Verification items for the finished model (mm, model axes). A direction names the side the tool comes from. Give positions to 0.01 mm unless a question says otherwise; leave off trailing zeros. Loops run counter-clockwise (first coordinate to the right, second up) from the corner with the lowest first, then second, coordinate; pieces in that order, holes last. Notation, with made-up numbers: (-10.5, -9) - (33.5, -9) arc R23 cw to (33.5, 9) - close; hole circle Ø5 at (-24.5, -1.5). An arc over 180 degrees is marked (long way). Use one line per item in the form item = value.
```python
from build123d import *

# Parameters (mm, degrees)
BOSS_EXTRUDE1_DEPTH                        = 1.6
CHAMFER1_SIZE                              = 3
BOSS_EXTRUDE2_DEPTH                        = 11
CHAMFER2_SIZE                              = 3
FILLET1_R                                  = 2
SKETCH3_R                                  = 1
CUT_EXTRUDE1_DEPTH                         = 11
SKETCH4_R                                  = 1.05
CUT_EXTRUDE2_DEPTH                         = 13.6
SKETCH5_R                                  = 1
CUT_EXTRUDE3_DEPTH                         = 2.6
MIRROR1_AT_THE_SECOND_PLANE_COPY_1_SKETC_R = 1
MIRROR1_AT_THE_SECOND_PLANE_COPY_1_DEPTH   = 11
MIRROR1_AT_THE_SECOND_PLANE_COPY_2_SKETC_R = 1.05
MIRROR1_AT_THE_SECOND_PLANE_COPY_2_DEPTH   = 13.6
MIRROR1_AT_THE_SECOND_PLANE_COPY_3_SKETC_R = 1
MIRROR1_AT_THE_SECOND_PLANE_COPY_3_DEPTH   = 2.6
SKETCH6_W                                  = 8.5
SKETCH6_H                                  = 7
BOSS_EXTRUDE3_DEPTH                        = 3.3
SKETCH7_R                                  = 0.5
SKETCH7_R_2                                = 1
CUT_EXTRUDE4_DEPTH                         = 2.6
LPATTERN1_COUNT                            = 3
LPATTERN1_PITCH                            = 2.54
LPATTERN1_COL_COUNT                        = 3
LPATTERN1_COL_PITCH                        = 2.54


with BuildPart() as part:
    # Sketch1 → Boss-Extrude1 (new body)
    with BuildSketch(Plane(origin=(0, 0, 0), x_dir=(1, 0, 0), z_dir=(0, 1, 0))):
        Polygon((-17, 20), (-17, -20), (17, -20), align=None)
        Polygon((17, 20), (17, -20), (-17, 20), align=None)
    extrude(amount=BOSS_EXTRUDE1_DEPTH)

    # Chamfer1
    chamfer1_edges = [part.edges().sort_by_distance(p)[0] for p in [
        (-17, 0.8, -20),
        (17, 0.8, -20),
        (17, 0.8, 20),
        (-17, 0.8, 20),
    ]]
    chamfer(chamfer1_edges, length=CHAMFER1_SIZE)

    # Sketch2 → Boss-Extrude2 (add)
    with BuildSketch(Plane(origin=(0, 1.6, 0), x_dir=(1, 0, 0), z_dir=(0, 1, 0))):
        Polygon((-15, 13), (15, 13), (15, -13), align=None)
        Polygon((-15, 13), (15, -13), (-15, -13), align=None)
    extrude(amount=BOSS_EXTRUDE2_DEPTH)

    # Chamfer2
    chamfer2_edges = [part.edges().sort_by_distance(p)[0] for p in [
        (15, 7.1, -13),
        (-15, 7.1, -13),
        (-15, 7.1, 13),
        (15, 7.1, 13),
    ]]
    chamfer(chamfer2_edges, length=CHAMFER2_SIZE)

    # Fillet1
    fillet1_edges = [part.edges().sort_by_distance(p)[0] for p in [
        (-15, 7.1, 10),
        (-15, 7.1, -10),
        (12, 7.1, -13),
        (-12, 7.1, -13),
        (15, 7.1, 10),
        (15, 7.1, -10),
        (-12, 7.1, 13),
        (12, 7.1, 13),
    ]]
    fillet(fillet1_edges, radius=FILLET1_R)

    # Sketch3 → Cut-Extrude1 (cut)
    with BuildSketch(Plane(origin=(0, 12.6, 0), x_dir=(1, 0, 0), z_dir=(0, 1, 0))):
        with Locations((-11.378679656, 9.378679656)):
            Circle(SKETCH3_R)
    cut_extrude1 = extrude(amount=-CUT_EXTRUDE1_DEPTH, mode=Mode.SUBTRACT)

    # Sketch4 → Cut-Extrude2 (cut, through all)
    with BuildSketch(Plane(origin=(0, 12.6, 0), x_dir=(1, 0, 0), z_dir=(0, 1, 0))):
        with Locations((15, 15.5)):
            Circle(SKETCH4_R)
    cut_extrude2 = extrude(amount=-CUT_EXTRUDE2_DEPTH, mode=Mode.SUBTRACT)

    # Sketch5 → Cut-Extrude3 (cut, through all)
    with BuildSketch(Plane(origin=(0, 1.6, 0), x_dir=(1, 0, 0), z_dir=(0, 1, 0))):
        with Locations((-12.35, 20)):
            Circle(SKETCH5_R)
    cut_extrude3 = extrude(amount=-CUT_EXTRUDE3_DEPTH, mode=Mode.SUBTRACT)

    # Mirror1: Cut-Extrude1, Cut-Extrude2, Cut-Extrude3 across plane
    add(cut_extrude1.mirror(Plane.XY), mode=Mode.SUBTRACT)
    add(cut_extrude2.mirror(Plane.XY), mode=Mode.SUBTRACT)
    add(cut_extrude3.mirror(Plane.XY), mode=Mode.SUBTRACT)

    # Mirror1 at the second plane: Cut-Extrude3, Cut-Extrude1, Cut-Extrude2 across plane
    add(cut_extrude3.mirror(Plane(origin=(0, 0, 0), x_dir=(0, 0, 1), z_dir=(1, 0, 0))), mode=Mode.SUBTRACT)
    add(cut_extrude1.mirror(Plane(origin=(0, 0, 0), x_dir=(0, 0, 1), z_dir=(1, 0, 0))), mode=Mode.SUBTRACT)
    add(cut_extrude2.mirror(Plane(origin=(0, 0, 0), x_dir=(0, 0, 1), z_dir=(1, 0, 0))), mode=Mode.SUBTRACT)

    # Mirror1 at the second plane copy 1 sketc → Mirror1 at the second plane copy 1 (cut)
    with BuildSketch(Plane(origin=(0, 12.6, 0), x_dir=(-1, 0, 0), z_dir=(0, 1, 0))):
        with Locations((-11.378679656, 9.378679656)):
            Circle(MIRROR1_AT_THE_SECOND_PLANE_COPY_1_SKETC_R)
    extrude(amount=-MIRROR1_AT_THE_SECOND_PLANE_COPY_1_DEPTH, mode=Mode.SUBTRACT)

    # Mirror1 at the second plane copy 2 sketc → Mirror1 at the second plane copy 2 (cut, through all)
    with BuildSketch(Plane(origin=(0, 12.6, 0), x_dir=(-1, 0, 0), z_dir=(0, 1, 0))):
        with Locations((15, 15.5)):
            Circle(MIRROR1_AT_THE_SECOND_PLANE_COPY_2_SKETC_R)
    extrude(amount=-MIRROR1_AT_THE_SECOND_PLANE_COPY_2_DEPTH, mode=Mode.SUBTRACT)

    # Mirror1 at the second plane copy 3 sketc → Mirror1 at the second plane copy 3 (cut, through all)
    with BuildSketch(Plane(origin=(0, 1.6, 0), x_dir=(-1, 0, 0), z_dir=(0, 1, 0))):
        with Locations((-12.35, 20)):
            Circle(MIRROR1_AT_THE_SECOND_PLANE_COPY_3_SKETC_R)
    extrude(amount=-MIRROR1_AT_THE_SECOND_PLANE_COPY_3_DEPTH, mode=Mode.SUBTRACT)

    # Sketch6 → Boss-Extrude3 (add)
    with BuildSketch(Plane(origin=(0, 1.6, 0), x_dir=(1, 0, 0), z_dir=(0, 1, 0))):
        with Locations((5.85, -16.5)):
            Rectangle(SKETCH6_W, SKETCH6_H)
    extrude(amount=BOSS_EXTRUDE3_DEPTH)

    # Sketch7 → Cut-Extrude4 (cut, through all)
    with BuildSketch(Plane(origin=(0, 1.6, 0), x_dir=(1, 0, 0), z_dir=(0, 1, 0))):
        with Locations((0, 18)):
            Circle(SKETCH7_R)
        with Locations((0, 20)):
            Circle(SKETCH7_R_2)
    cut_extrude4 = extrude(amount=-CUT_EXTRUDE4_DEPTH, mode=Mode.SUBTRACT)

    # LPattern1: Cut-Extrude4 ×3
    with Locations(*[(i * LPATTERN1_PITCH, 0, 0) for i in range(1, LPATTERN1_COUNT)]):
        add(cut_extrude4, mode=Mode.SUBTRACT)

    # LPattern1 col: Cut-Extrude4 ×3
    with Locations(*[(-i * LPATTERN1_COL_PITCH, 0, 0) for i in range(1, LPATTERN1_COL_COUNT)]):
        add(cut_extrude4, mode=Mode.SUBTRACT)


solid = part.part
```
1. Scan lines: probe 1 along Z at (x, y) = (-15, 0.7); probe 2 along X at (y, z) = (5.25, -10); probe 3 along X at (y, z) = (6.5, -9). Record each from-to range of solid material in increasing order.
Result set:
probe_1 = -19 to -16.55, -14.45 to 14.45, 16.55 to 19
probe_2 = -14.82 to -12.16, -10.6 to 10.6, 12.16 to 14.82
probe_3 = -15 to -12.3, -10.45 to 10.45, 12.3 to 15
2. Section check A-A, the plane x = 5.08. Record the cut outline in (y, z).
Result set:
outline = (0, -19) - (1.6, -19) - (1.6, -18.5) - (0, -18.5) - close; (0, -17.5) - (1.6, -17.5) - (1.6, -13) - (12.6, -13) - (12.6, 13) - (4.9, 13) - (4.9, 20) - (0, 20) - close
3. Section check D-D, the plane y = 11.75. Record the cut outline in (x, z), then the cut area to 3 significant figures.
Result set:
outline = (-15, -9.17) arc R2 ccw to (-14.41, -10.59) - (-12.59, -12.41) arc R2 ccw to (-11.17, -13) - (11.17, -13) arc R2 ccw to (12.59, -12.41) - (14.41, -10.59) arc R2 ccw to (15, -9.17) - (15, 9.17) arc R2 ccw to (14.41, 10.59) - (12.59, 12.41) arc R2 ccw to (11.17, 13) - (-11.17, 13) arc R2 ccw to (-12.59, 12.41) - (-14.41, 10.59) arc R2 ccw to (-15, 9.17) - close; hole circle Ø2 at (-11.38, -9.38); hole circle Ø2 at (-11.38, 9.38); hole circle Ø2 at (11.38, -9.38); hole circle Ø2 at (11.38, 9.38)
area = 749 mm²
4. Tool access check on faces 4 (the flat face through (-13, 7, 12)), 5 (the flat face through (6, 4.9, 16)), 6 (the flat face through (11, 1.6, 9)). Record the directions out of +Z, -Z, +X, -X, +Y, -Y that give a thin tool (end or side, any length) a straight path to the whole face; none if there is none.
Result set:
face_4 = +Z, -X, +Y
face_5 = +Z, +X, -X, +Y
face_6 = +Y
5. Draft check along Z on faces 1 (the flat face through (-4, 1.6, -14)), 2 (the cylindrical face through (-5.1, 0.8, -18.5)), 3 (the flat face through (-13, 7, -12)). Enter one of: released by +Z, released by -Z, zero draft, split by the parting line, or undercut.
Result set:
face_1 = zero draft
face_2 = undercut
face_3 = released by -Z
6. Section check C-C, the plane x = 8.5. Record the cut outline in (y, z).
Result set:
outline = (0, -20) - (1.6, -20) - (1.6, -13) - (12.6, -13) - (12.6, 13) - (4.9, 13) - (4.9, 20) - (0, 20) - close
7. Depth check by flat-ended pin: pin 1 Ø2 at (x, z) = (7, 15.5) entering from +Y; pin 2 Ø4 at (y, z) = (8, -9) entering from +X; pin 3 Ø1 at (y, z) = (9.5, 12) entering from -X; pin 4 Ø1.9 at (x, z) = (-15, -15.5) entering from -Y (3 decimals). Enter the tip coordinate at first touch or a pass-through.
Result set:
pin_1 = 4.9
pin_2 = 15
pin_3 = -13.5
pin_4 = through
8. Section check B-B, the plane z = -15.5. Record the cut outline in (x, y).
Result set:
outline = (-17, 0) - (-16.05, 0) - (-16.05, 1.6) - (-17, 1.6) - close; (-13.95, 0) - (13.95, 0) - (13.95, 1.6) - (-13.95, 1.6) - close; (16.05, 0) - (17, 0) - (17, 1.6) - (16.05, 1.6) - close
